Input: dimensioned drawing with shaded views. Units: mm. Origin: part minimum x, y, z. A direction names the side the tool comes from. Give positions to 0.01 mm unless a question says otherwise; leave off trailing zeros. Loops run counter-clockwise (first coordinate to the right, second up) from the corner with the lowest first, then second, coordinate; pieces in that order, holes last. Notation, with made-up numbers: M -2,7.25 L 43,7.25 A18 cw 43,39.25 Z; hole C -32.5,15 d11. An arc over 180 degrees is marked long. Use CSV: the item, a comma, the result in double quotes. Start each with the question number.
Q1. Reachability of the marked faces 1 and 2 from +Z, -Z, +X, -X, +Y, -Y: full face, straight path, thin tool, end or side. Return the list, or none.
Q2. Section C-C, the plane y = 12.5. Output: boundary loops of the cut face in (x, z), plus the area to 3 significant figures.
Q3. Section D-D, the plane z = 48. Output: boundary loops of the cut face in (x, y), plus the area to 3 significant figures.
Q4. Section B-B, the plane z = 15.5. Output: boundary loops of the cut face in (x, y), plus the area to 3 significant figures.
Q5. Material intervals for line 1 along Z through (x, y) = (15, 14.75); line 2 along Z through (x, y) = (15.25, 21.75); line 3 along Y through (x, z) = (4, 16.2), sorted ascending.
Q6. Pin query (flat end, axial travel): pin 1 (4 mm diameter, centred on x = 12.5, y = 19.5, fed in from -Z); pin 2 (1.5 mm diameter, centred on x = 12.5, y = 4, fed in from +Z); pin 3 (7.5 mm diameter, centred on x = 18, y = 17, fed in from -Z). Return the tip coordinate at first contact, or that it passes through.
Q7. Section A-A, the plane x = 12.5. Output: boundary loops of the cut face in (y, z).
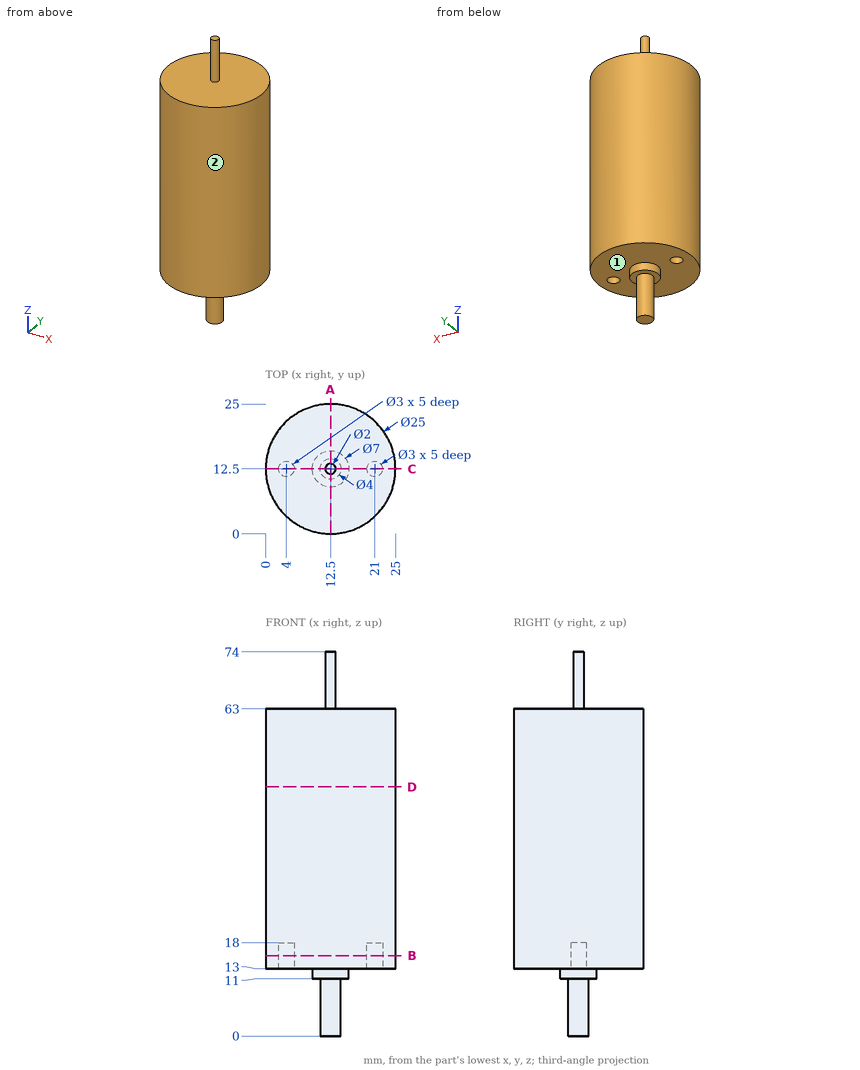
A:
1,face 1,"-Z"
1,face 2,"+Z, -Z"
2,outline,"M 0,13 L 2.5,13 L 2.5,18 L 5.5,18 L 5.5,13 L 9,13 L 9,11 L 10.5,11 L 10.5,0 L 14.5,0 L 14.5,11 L 16,11 L 16,13 L 19.5,13 L 19.5,18 L 22.5,18 L 22.5,13 L 25,13 L 25,63 L 13.5,63 L 13.5,74 L 11.5,74 L 11.5,63 L 0,63 Z"
2,area,"1,300 mm^2"
3,outline,"C 12.5,12.5 d25"
3,area,"491 mm^2"
4,outline,"C 12.5,12.5 d25; hole C 4,12.5 d3; hole C 21,12.5 d3"
4,area,"477 mm^2"
5,line 1,"11 to 63"
5,line 2,"13 to 63"
5,line 3,"3.33 to 11, 14 to 21.67"
6,pin 1,"z = 13"
6,pin 2,"z = 63"
6,pin 3,"z = 11"
7,outline,"M 0,13 L 9,13 L 9,11 L 10.5,11 L 10.5,0 L 14.5,0 L 14.5,11 L 16,11 L 16,13 L 25,13 L 25,63 L 13.5,63 L 13.5,74 L 11.5,74 L 11.5,63 L 0,63 Z"
